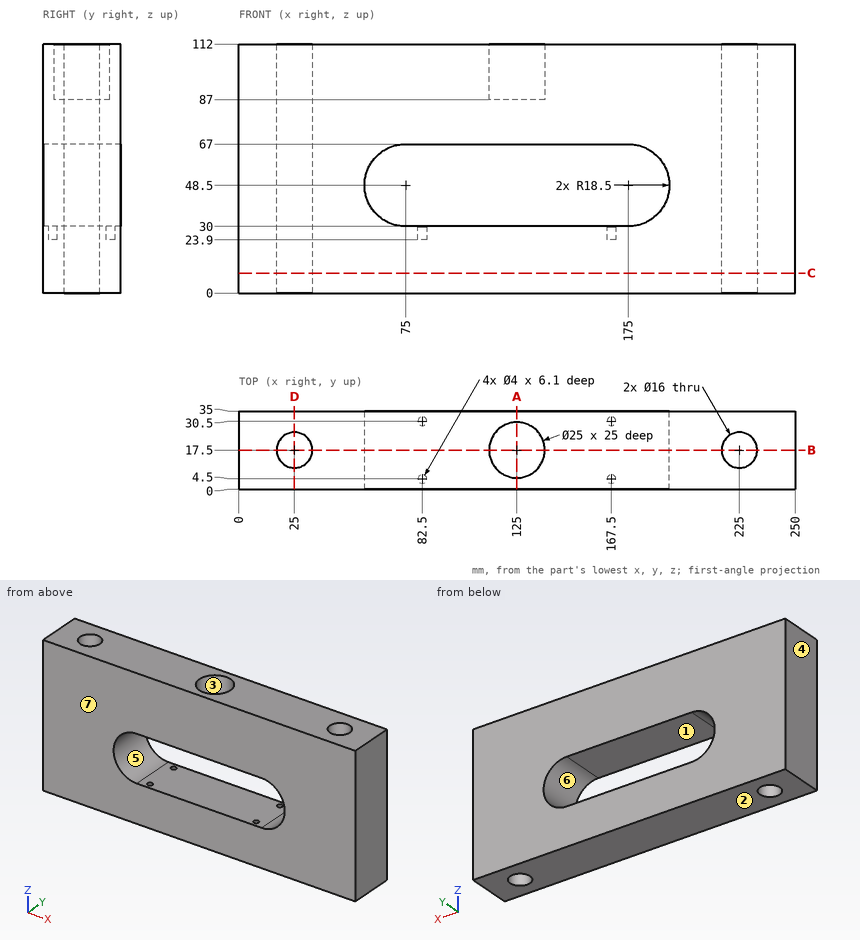
Can you work these out from the drawing? Everything is in mm from the part's minimum corner. A direction names the side the tool comes from. Coordinates: 2 decimals unless noted, no trailing zeros. Order: outer loops, then holes, each group sorted by start corner. A loop starts at its lowest first (then second) coordinate and runs counter-clockwise, first axis right, second up. Notation, with made-up numbers: M -7.5,35.5 L 46.5,35.5 A24 cw 46.5,50.5 Z; hole C 55,47.25 d1. An arc over 180 degrees is marked long. Answer as CSV lines item,"result". Start each with the question number.
1. I want a section at D-D, the plane x = 25. Write out the boundary of the cut face in (y, z), and give its area (3 significant figures).
2. We'd pull the mould along X, two halves only. Please class the marked faces 4, 5, 6 and 7: released by +X, released by -X, zero draft, split by the parting line, or undercut.
3. I want a section at A-A, the plane x = 125. Write out the boundary of the cut face in (y, z).
4. For pin 1 (12.5 mm diameter, centred on x = 127.5, y = 20, fed in from +Z), with a flat end and sliding along its axis, tell me the tip position at first contact or that it passes through.
5. On a 3-axis mill with a long thin cutter (end or side, diameter ignored), from which of +Z, -Z, +X, -X, +Y, -Y can I reach the whole of each face in a straight line? I mean the marked faces 1, 2 and 3. Say none if no direction works.
6. I want a section at C-C, the plane z = 9. Write out the boundary of the cut face in (x, y), and give its area (3 significant figures).
7. I want a section at B-B, the plane y = 17.5. Write out the boundary of the cut face in (x, z).
8. I need wall thicknesses on line 1 (Y direction, x = 167.5, z = 27.75); line 2 (Z direction, x = 120.5, y = 7); line 3 (Y direction, x = 167, z = 25). Which ranges of each line are inside material? Lowest first, please. Write a range as [from, to].
Recorded:
1,outline,"M 0,0 L 9.5,0 L 9.5,112 L 0,112 Z; M 25.5,0 L 35,0 L 35,112 L 25.5,112 Z"
1,area,"2,130 mm2"
2,face 4,"released by -X"
2,face 5,"undercut"
2,face 6,"undercut"
2,face 7,"zero draft"
3,outline,"M 0,0 L 35,0 L 35,30 L 0,30 Z; M 0,67 L 35,67 L 35,112 L 30,112 L 30,87 L 5,87 L 5,112 L 0,112 Z"
4,pin 1,"stops at z = 87"
5,face 1,"+Y, -Y"
5,face 2,"-Z, +X, -X, +Y, -Y"
5,face 3,"+Z"
6,outline,"M 0,0 L 250,0 L 250,35 L 0,35 Z; hole C 25,17.5 d16; hole C 225,17.5 d16"
6,area,"8,350 mm2"
7,outline,"M 0,0 L 17,0 L 17,112 L 0,112 Z; M 33,0 L 217,0 L 217,112 L 137.5,112 L 137.5,87 L 112.5,87 L 112.5,112 L 33,112 Z; M 233,0 L 250,0 L 250,112 L 233,112 Z; hole M 75,30 L 175,30 A18.5 ccw 175,67 L 75,67 A18.5 ccw Z"
8,line 1,"y = [0, 2.5], [6.5, 28.5], [32.5, 35]"
8,line 2,"z = [0, 30], [67, 87]"
8,line 3,"y = [0, 2.56], [6.44, 28.56], [32.44, 35]"
